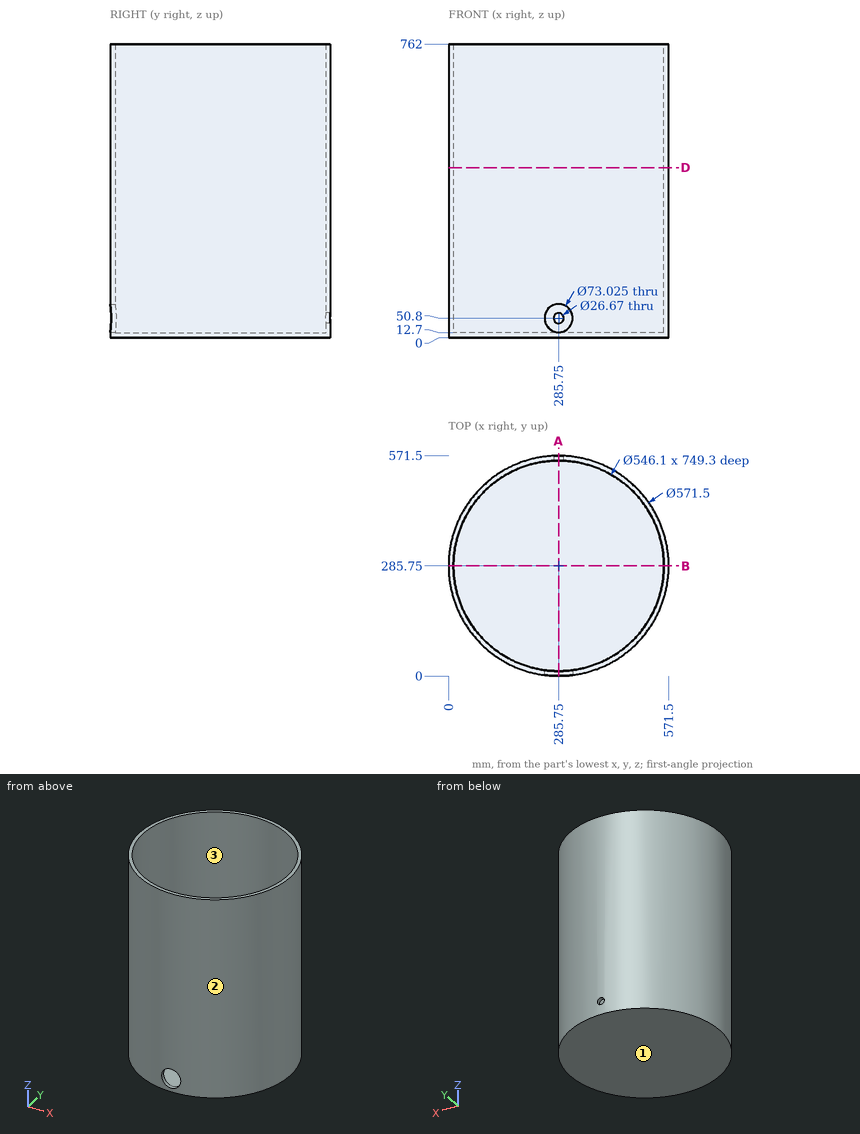
Design review of the part shown in the three views and the two pictorial views. Dimensions are in mm from the part's minimum x, y and z. Round coordinates to 2 decimals unless told otherwise and drop trailing zeros. Loops run counter-clockwise (first coordinate to the right, second up) from the corner with the lowest first, then second, coordinate; pieces in that order, holes last. Notation, with made-up numbers: M 2.5,8 L 8.5,8 A16 cw 8.5,26 Z; hole C -8,52 d9. An arc over 180 degrees is marked long. Write item = value, one per line.
Item 1: Take a section at B-B on y = 285.75. Write out the cut boundary in (x, z), then the cut area to 3 significant figures.
Return value:
outline = M 0,0 L 571.5,0 L 571.5,762 L 558.8,762 L 558.8,12.7 L 12.7,12.7 L 12.7,762 L 0,762 Z
area = 26,300 mm2
Item 2: Take a section at A-A on x = 285.75. Write out the cut boundary in (y, z) (1 decimal), then the cut area to 3 significant figures.
Return value:
outline = M 0,0 L 571.5,0 L 571.5,37.5 L 558.8,37.5 L 558.8,12.7 L 12.7,12.7 L 12.7,14.3 L 0,14.3 Z; M 0,87.3 L 12.7,87.3 L 12.7,762 L 0,762 Z; M 558.8,64.1 L 571.5,64.1 L 571.5,762 L 558.8,762 Z
area = 25,000 mm2
Item 3: Take a section at D-D on z = 441. Write out the cut boundary in (x, y), then the cut area to 3 significant figures.
Return value:
outline = C 285.75,285.75 d571.5; hole C 285.75,285.75 d546.1
area = 22,300 mm2
Item 4: The part is to be moulded in two halves that separate along X. For the marked faces 1, 2 and 3, say which applies: released by +X, released by -X, zero draft, split by the parting line, or undercut.
Return value:
face_1 = zero draft
face_2 = split by the parting line
face_3 = undercut
Item 5: Insertion check: P1, Ø4, axis at y = 397.5, z = 334, coming from the +X side; P2, Ø10, axis at x = 239, z = 399.5, coming from the +Y side; P3, Ø3, axis at x = 119.5, z = 164, coming from the -Y side. Each pin has a flat end and moves straight along its axis. Give the tip position at first contact, or say it passes through.
Return value:
P1 = 549.58
P2 = 568.43
P3 = 52.28
Item 6: For line 1 (Y direction, x = 285, z = 528); line 2 (Z direction, x = 285.75, y = 5.25); line 3 (X direction, y = 311.5, z = 661), list the stretches that pass through material, from the lowest coordinate up. Write a range as [from, to].
Return value:
line_1 = [0, 12.7], [558.8, 571.5]
line_2 = [0, 14.29], [87.31, 762]
line_3 = [1.16, 13.92], [557.58, 570.34]
